Work out the finished part from the listing and answer in its coordinate system (mm). Face numbers are marked on the shaded views. Give positions to 0.01 mm unless a question says otherwise; leave off trailing zeros. Order: outer loops, then holes, each group sorted by start corner. A loop starts at its lowest first (then second) coordinate and runs counter-clockwise, first axis right, second up. Notation, with made-up numbers: (44, 0.25) - (98, 0.25) arc R9 cw to (98, 14.25) - close; hole circle Ø11 at (20.25, 31). An arc over 180 degrees is marked (long way). Write each question's results on one line, items separated by ' | '.
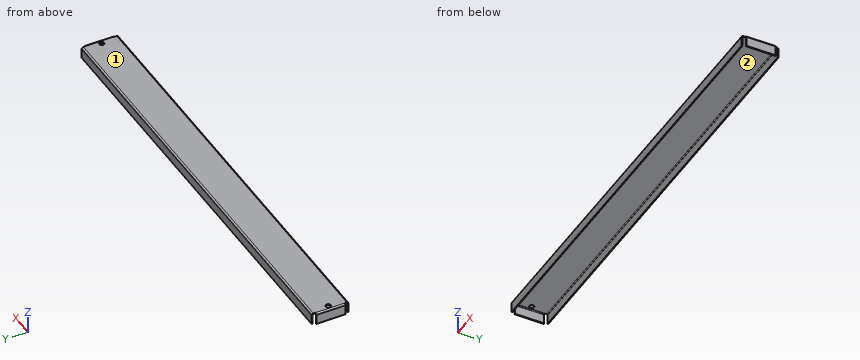
from build123d import *

# Parameters (mm, degrees)
CROQUIS1_W                   = 731.774
CROQUIS1_H                   = 61.976
BRIDA_BASE1_DEPTH            = 1.524
CROQUIS6_W                   = 3.1242
CROQUIS6_H                   = 6.35
CORTAR_EXTRUIR1_DEPTH        = 368.200048324
BRIDA_START                  = -362.7628
BRIDA_DE_ARISTA1_DEPTH       = 725.5256
BRIDA_START_2                = 6.35
BRIDA_DE_ARISTA1_2_DEPTH     = 49.276
BRIDA_DE_ARISTA1_3_DEPTH     = 725.5256
BRIDA_DE_ARISTA1_4_OUTLINE_W = 0.1524
BRIDA_DE_ARISTA1_4_OUTLINE_H = 1.524
BRIDA_DE_ARISTA1_4_DEPTH     = 0.0762
BRIDA_START_3                = 362.6866
BRIDA_DE_ARISTA1_5_OUTLINE_W = 0.1524
BRIDA_DE_ARISTA1_5_OUTLINE_H = 1.524
BRIDA_DE_ARISTA1_5_DEPTH     = 0.0762
BRIDA_DE_ARISTA1_6_DEPTH     = 49.276
CROQUIS19_R                  = 3.9624
CORTAR_EXTRUIR2_DEPTH        = 368.690706183


# Read off the part's stored shape, not the designer's step: Brida de arista1
# Sheet-metal steps are written as plain solids
with BuildPart() as part:
    # Croquis1 → Brida base1 (new body)
    with BuildSketch(Plane.XY):
        Rectangle(CROQUIS1_W, CROQUIS1_H)
    extrude(amount=-BRIDA_BASE1_DEPTH)

    # Croquis6 → Cortar-Extruir1 (cut, through all)
    with BuildSketch(Plane.XY):
        with Locations((364.3249, 27.813)):
            Rectangle(CROQUIS6_W, CROQUIS6_H)
        with Locations((364.3249, -27.813)):
            Rectangle(CROQUIS6_W, CROQUIS6_H)
        with Locations((-364.3249, -27.813)):
            Rectangle(CROQUIS6_W, CROQUIS6_H)
        with Locations((-364.3249, 27.813)):
            Rectangle(CROQUIS6_W, CROQUIS6_H)
    extrude(amount=-CORTAR_EXTRUIR1_DEPTH, mode=Mode.SUBTRACT)

    # Brida de arista1 outline → Brida de arista1 (add)
    with BuildSketch(Plane.YZ.offset(BRIDA_START)):
        with BuildLine():
            Line((30.988, -19.05), (30.988, -3.048))
            ThreePointArc((30.988, -3.048), (30.884141918, -2.259119551), (30.579645431, -1.524))
            Line((30.579645431, -1.524), (27.94, -1.524))
            ThreePointArc((27.94, -1.524), (29.017630735, -1.970369265), (29.464, -3.048))
            Line((29.464, -3.048), (29.464, -19.05))
            Line((29.464, -19.05), (30.988, -19.05))
        make_face()
        with BuildLine():
            ThreePointArc((-29.464, -3.048), (-29.017630735, -1.970369265), (-27.94, -1.524))
            Line((-27.94, -1.524), (-30.579645431, -1.524))
            ThreePointArc((-30.579645431, -1.524), (-30.884141918, -2.259119551), (-30.988, -3.048))
            Line((-30.988, -3.048), (-30.988, -19.05))
            Line((-30.988, -19.05), (-29.464, -19.05))
            Line((-29.464, -19.05), (-29.464, -3.048))
        make_face()
    extrude(amount=BRIDA_DE_ARISTA1_DEPTH)

    # Brida de arista1 2 outline → Brida de arista1 2 (add)
    with BuildSketch(Plane(origin=(0, 30.988, -1.524), x_dir=(-1, 0, 0), z_dir=(0, -1, 0)).offset(BRIDA_START_2)):
        with BuildLine():
            Line((-364.363, 1.524), (-364.363, 17.526))
            Line((-364.363, 17.526), (-365.887, 17.526))
            Line((-365.887, 17.526), (-365.887, 1.524))
            ThreePointArc((-365.887, 1.524), (-365.783141918, 0.735119551), (-365.478645431, 0))
            Line((-365.478645431, 0), (-362.839, 0))
            ThreePointArc((-362.839, 0), (-363.916630735, 0.446369265), (-364.363, 1.524))
        make_face()
        with BuildLine():
            ThreePointArc((364.363, 1.524), (363.916630735, 0.446369265), (362.839, 0))
            Line((362.839, 0), (365.478645431, 0))
            ThreePointArc((365.478645431, 0), (365.783141918, 0.735119551), (365.887, 1.524))
            Line((365.887, 1.524), (365.887, 17.526))
            Line((365.887, 17.526), (364.363, 17.526))
            Line((364.363, 17.526), (364.363, 1.524))
        make_face()
    extrude(amount=BRIDA_DE_ARISTA1_2_DEPTH)

    # Brida de arista1 3 outline → Brida de arista1 3 (cut)
    with BuildSketch(Plane.YZ.offset(BRIDA_START)):
        with BuildLine():
            ThreePointArc((27.94, 0), (29.464, -0.408354569), (30.579645431, -1.524))
            Line((30.579645431, -1.524), (30.988, -1.524))
            Line((30.988, -1.524), (30.988, 0))
            Line((30.988, 0), (27.94, 0))
        make_face()
        with BuildLine():
            ThreePointArc((-30.579645431, -1.524), (-29.464, -0.408354569), (-27.94, 0))
            Line((-27.94, 0), (-30.988, 0))
            Line((-30.988, 0), (-30.988, -1.524))
            Line((-30.988, -1.524), (-30.579645431, -1.524))
        make_face()
    extrude(amount=BRIDA_DE_ARISTA1_3_DEPTH, mode=Mode.SUBTRACT)

    # Brida de arista1 4 outline → Brida de arista1 4 (cut)
    with BuildSketch(Plane.YZ.offset(BRIDA_START)):
        with Locations((24.7142, -0.762)):
            Rectangle(BRIDA_DE_ARISTA1_4_OUTLINE_W, BRIDA_DE_ARISTA1_4_OUTLINE_H)
        with Locations((-24.7142, -0.762)):
            Rectangle(BRIDA_DE_ARISTA1_4_OUTLINE_W, BRIDA_DE_ARISTA1_4_OUTLINE_H)
    extrude(amount=BRIDA_DE_ARISTA1_4_DEPTH, mode=Mode.SUBTRACT)

    # Brida de arista1 5 outline → Brida de arista1 5 (cut)
    with BuildSketch(Plane.YZ.offset(BRIDA_START_3)):
        with Locations((24.7142, -0.762)):
            Rectangle(BRIDA_DE_ARISTA1_5_OUTLINE_W, BRIDA_DE_ARISTA1_5_OUTLINE_H)
        with Locations((-24.7142, -0.762)):
            Rectangle(BRIDA_DE_ARISTA1_5_OUTLINE_W, BRIDA_DE_ARISTA1_5_OUTLINE_H)
    extrude(amount=BRIDA_DE_ARISTA1_5_DEPTH, mode=Mode.SUBTRACT)

    # Brida de arista1 6 outline → Brida de arista1 6 (cut)
    with BuildSketch(Plane(origin=(0, 30.988, -1.524), x_dir=(-1, 0, 0), z_dir=(0, -1, 0)).offset(BRIDA_START_2)):
        with BuildLine():
            ThreePointArc((-362.839, -1.524), (-364.363, -1.115645431), (-365.478645431, 0))
            Line((-365.478645431, 0), (-365.887, 0))
            Line((-365.887, 0), (-365.887, -1.524))
            Line((-365.887, -1.524), (-362.839, -1.524))
        make_face()
        with BuildLine():
            Line((365.887, 0), (365.478645431, 0))
            ThreePointArc((365.478645431, 0), (364.363, -1.115645431), (362.839, -1.524))
            Line((362.839, -1.524), (365.887, -1.524))
            Line((365.887, -1.524), (365.887, 0))
        make_face()
    extrude(amount=BRIDA_DE_ARISTA1_6_DEPTH, mode=Mode.SUBTRACT)

    # Croquis19 → Cortar-Extruir2 (cut, through all)
    with BuildSketch(Plane.XY):
        with Locations((-357.251, 0)):
            Circle(CROQUIS19_R)
        with Locations((357.251, 0)):
            Circle(CROQUIS19_R)
    extrude(amount=-CORTAR_EXTRUIR2_DEPTH, mode=Mode.SUBTRACT)


solid = part.part
1. Determine the mould class of the marked faces 1 and 2 for opening direction Y: +Y half, -Y half, draft (parallel to the pull), parting line (faces both ways), or undercut.
Answer list:
face 1: draft | face 2: undercut
2. A cutting plane is placed at A-A, the plane z = -6.25. Write down the section's boundary in (x, y).
Answer list:
outline: (-365.89, -24.64) - (-364.36, -24.64) - (-364.36, 24.64) - (-365.89, 24.64) - close; (-362.76, -30.99) - (362.76, -30.99) - (362.76, -29.46) - (-362.76, -29.46) - close; (-362.76, 29.46) - (362.76, 29.46) - (362.76, 30.99) - (-362.76, 30.99) - close; (364.36, -24.64) - (365.89, -24.64) - (365.89, 24.64) - (364.36, 24.64) - close
3. A cutting plane is placed at B-B, the plane x = 269.5. Write down the section's boundary in (y, z).
Answer list:
outline: (-30.99, -19.05) - (-29.46, -19.05) - (-29.46, -3.05) arc R1.52 cw to (-27.94, -1.52) - (27.94, -1.52) arc R1.52 cw to (29.46, -3.05) - (29.46, -19.05) - (30.99, -19.05) - (30.99, -3.05) arc R3.05 ccw to (27.94, 0) - (-27.94, 0) arc R3.05 ccw to (-30.99, -3.05) - close
4. Straight lines are drawn through the part: line 1 (X direction, y = 7, z = -7.25); line 2 (Y direction, x = -102, z = -7.5); line 3 (Z direction, x = -249.5, y = -17). For each, find the intervals that lie inside material, in ascending order. Write a range as [from, to].
Answer list:
line 1: [-365.89, -364.36], [364.36, 365.89] | line 2: [-30.99, -29.46], [29.46, 30.99] | line 3: [-1.52, 0]
5. Given P1, Ø1.9, axis at y = -27.5, z = -10, coming from the +X side; P2, Ø1.5, axis at x = -134, y = 13, coming from the -Z side; P3, Ø7, axis at y = 28.5, z = -13, coming from the +X side; P4, Ø5, axis at y = 27.5, z = -10, coming from the -X side, each flat-ended and moving along its own axis, determine where each tip first touches the part or whether it passes through.
Answer list:
P1: through | P2: z = -1.52 | P3: x = 362.76 | P4: x = -362.76
6. A cutting plane is placed at C-C, the plane y = -18. Write down the section's boundary in (x, z).
Answer list:
outline: (-365.89, -19.05) - (-364.36, -19.05) - (-364.36, -3.05) arc R1.52 cw to (-362.84, -1.52) - (362.84, -1.52) arc R1.52 cw to (364.36, -3.05) - (364.36, -19.05) - (365.89, -19.05) - (365.89, -3.05) arc R3.05 ccw to (362.84, 0) - (-362.84, 0) arc R3.05 ccw to (-365.89, -3.05) - close
